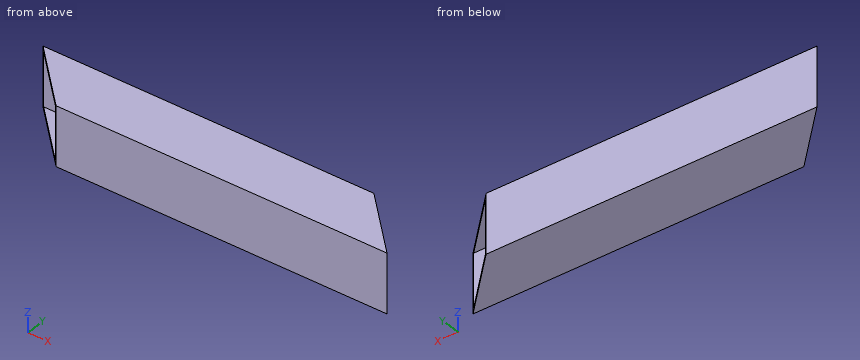
```python
from build123d import *

# Parameters (mm, degrees)
F0_W     = 232
F0_H     = 50
F1_DEPTH = 50
F2_T     = -2.54


with BuildPart() as f1:
    # F0 (on Top) → F1 (new body)
    with BuildSketch(Plane.XY):
        Rectangle(F0_W, F0_H)
        Polygon((-166, 25), (-116, -25), (-116, 25), align=None)
        Polygon((116, 25), (116, -25), (166, -25), align=None)
    extrude(amount=F1_DEPTH)

    # F2
    f2_openings = [f1.faces().sort_by_distance(p)[0] for p in [
        (-141, 0, 25),
        (141, 0, 25),
    ]]
    offset(amount=F2_T, openings=f2_openings)


solid = f1.part
```
Read the model definition and answer for the solid it produces. Units are mm, in the model's axes. Round coordinates to 2 decimals unless told otherwise and drop trailing zeros. Write each loop counter-clockwise with the first axis right and the second up, starting at its lowest first coordinate (ties: lowest second). Pieces come first, ordered by that corner, then holes. Notation, with made-up numbers: (82.25, -28.75) - (112.25, -28.75) arc R14 ccw to (112.25, -6.75) - close; hole circle Ø1 at (-24, 67). An arc over 180 degrees is marked (long way). Use CSV: the item, a comma, the result in double quotes.
Q1. This flat-tipped pin is pushed along its axis until it touches: pin 1 Ø10 at (y, z) = (13, 23) entering from +X. Where does it stop, or does it pass through?
Values:
pin 1,"passes through"
Q2. Straight lines are drawn through the part: line 1 along Y through (x, z) = (24, 36); line 2 along Z through (x, y) = (-80, 19); line 3 along Y through (x, z) = (-125.5, 35). For each, find the intervals that lie inside material, in ascending order.
Values:
line 1,"y = -25 to -22.46, 22.46 to 25"
line 2,"z = 0 to 2.54, 47.46 to 50"
line 3,"y = 22.46 to 25"
Q3. Find section B-B, the plane z = 22. Write down the section's boundary in (x, y), then the cut area to 3 significant figures.
Values:
outline,"(-166, 25) - (-163.46, 22.46) - (118.54, 22.46) - (116, 25) - close; (-118.54, -22.46) - (-116, -25) - (166, -25) - (163.46, -22.46) - close"
area,"1,430 mm²"
Q4. Find section A-A, the plane y = 2.5. Write down the section's boundary in (x, z).
Values:
outline,"(-143.5, 0) - (138.5, 0) - (138.5, 2.54) - (-143.5, 2.54) - close; (-143.5, 47.46) - (138.5, 47.46) - (138.5, 50) - (-143.5, 50) - close"
Q5. Find section C-C, the plane x = 43. Write down the section's boundary in (y, z).
Values:
outline,"(-25, 0) - (25, 0) - (25, 50) - (-25, 50) - close; hole (-22.46, 2.54) - (22.46, 2.54) - (22.46, 47.46) - (-22.46, 47.46) - close"
